Could you check a few things on this drawing? It's one solid part, dimensions in mm from its lowest x, y, z. A direction names the side the tool comes from. Give positions to 0.01 mm unless a question says otherwise; leave off trailing zeros. Loops run counter-clockwise (first coordinate to the right, second up) from the corner with the lowest first, then second, coordinate; pieces in that order, holes last. Notation, with made-up numbers: M 63,48 L 102,48 A12 ccw 102,57 Z; hole C -20.5,-3 d2. An arc over 180 degrees is marked long. Answer in a Markdown table with one row per item. Add a question column.
1. If we section it at D-D on y = 2.5: List the corners of the cut face in (x, z) for me.
2. If we section it at A-A on y = 16: List the corners of the cut face in (x, z) for me.
3. Which directions (+Z, -Z, +X, -X, +Y, -Y) give clear straight access to the entire face, cutting with the end or side of a thin tool? Please do the marked faces 1 and 2.
4. I'm going to push flat-ended pins straight in: pin 1 Ø9 at (x, y) = (21.75, 16) entering from -Z; pin 2 Ø3 at (x, y) = (24, 11.5) entering from +Z. Where does each tip first touch, or does it pass through?
5. If we section it at C-C on x = 21.75: List the corners of the cut face in (y, z) for me, then the cut area to 3 significant figures.
6. I need wall thicknesses on line 1 along Y through (x, z) = (42.8, 21.3); line 2 along X through (y, z) = (30.5, 18.5); line 3 along Z through (x, y) = (32.5, 24). Which ranges of each line are inside material? Lowest first, please. Write a range as from..to.
7. Thinking about a two-plate mould opening in X: for the marked faces 3, 4 and 5, which applies, released by +X, released by -X, zero draft, split by the parting line, or undercut?
8. If we section it at B-B on z = 14.5: List the corners of the cut face in (x, y) for me.
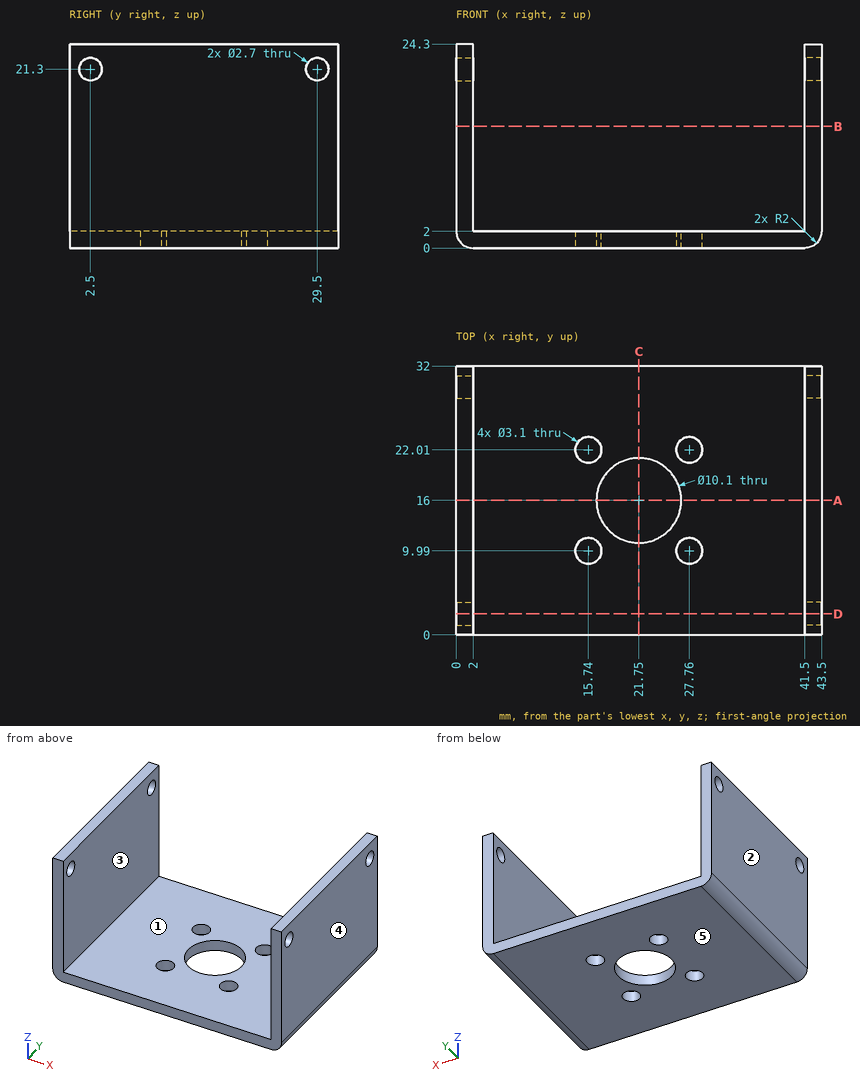
Results:
| question | item | result |
|---|---|---|
| 1 | outline | M 0,2 A2 ccw 2,0 L 41.5,0 A2 ccw 43.5,2 L 43.5,19.95 L 41.5,19.95 L 41.5,2 L 2,2 L 2,19.95 L 0,19.95 Z; M 0,22.65 L 2,22.65 L 2,24.3 L 0,24.3 Z; M 41.5,22.65 L 43.5,22.65 L 43.5,24.3 L 41.5,24.3 Z |
| 2 | outline | M 0,2 A2 ccw 2,0 L 16.7,0 L 16.7,2 L 2,2 L 2,24.3 L 0,24.3 Z; M 26.8,0 L 41.5,0 A2 ccw 43.5,2 L 43.5,24.3 L 41.5,24.3 L 41.5,2 L 26.8,2 Z |
| 3 | face 1 | +Z, +Y, -Y |
| 3 | face 2 | +Z, -Z, -X, +Y, -Y |
| 4 | pin 1 | through |
| 4 | pin 2 | z = 2 |
| 5 | outline | M 0,0 L 10.95,0 L 10.95,2 L 0,2 Z; M 21.05,0 L 32,0 L 32,2 L 21.05,2 Z |
| 5 | area | 43.8 mm2 |
| 6 | line 1 | 0..1.15, 3.85..28.15, 30.85..32 |
| 6 | line 2 | 0..2, 41.5..43.5 |
| 6 | line 3 | 0..2 |
| 7 | face 3 | undercut |
| 7 | face 4 | released by +X |
| 7 | face 5 | zero draft |
| 8 | outline | M 0,0 L 2,0 L 2,32 L 0,32 Z; M 41.5,0 L 43.5,0 L 43.5,32 L 41.5,32 Z |
